Check sheet for the modelled part. Datum: model origin and axes. Units: mm. Coordinates: 2 decimals unless noted, no trailing zeros. Order: outer loops, then holes, each group sorted by start corner. A loop starts at its lowest first (then second) coordinate and runs counter-clockwise, first axis right, second up. Notation, with made-up numbers: M 59,88.25 L 80,88.25 A20 cw 80,116.25 Z; hole C 70,83.5 d7. An arc over 180 degrees is marked long. Answer in a Markdown table with one row per item. Add a question column.
Autodesk Fusion 360 part; units mm, degrees
sketch "Sketch1" plane through (0, 0, 0) normal (0, 0, 1) x (1, 0, 0)
  line L0 (-11.375, 11.375) -> (11.375, 11.375)
  line L1 (11.375, 11.375) -> (11.375, -11.375)
  line L2 (11.375, -11.375) -> (-11.375, -11.375)
  line L3 (-11.375, -11.375) -> (-11.375, 11.375)
  circle A0 centre (0, 0) radius 9
  point P0 (0, 11.375)
  point P1 (11.375, 0)
  dimension "d1" = 22.75
  dimension "d2" = 18
extrude "Extrude3" add sketch "Sketch1" along normal blind 9.75
1. Section check B-B on z = 1.75. Enter the section's corners in (x, y) (3 decimals).
2. Release check for a two-part mould opening along X. For faces 1 (the flat face through (11.375, 0, 5)), 2 (the flat face through (-11.375, 0, 5)), 3 (the cylindrical face through (-1.172, -8.923, 4.807)), 4 (the flat face through (0, -11.375, 5)) record: released by +X, released by -X, zero draft, split by the parting line, or undercut.
3. Scan lines: line 1 (Y direction, x = 0, z = 3) (3 decimals); line 2 (Y direction, x = -1.5, z = 0.5) (3 decimals); line 3 (X direction, y = -5, z = 0.75) (3 decimals). Record each from-to range of solid material in increasing order.
4. Section check A-A on y = 0. Enter the section's corners in (x, z) (3 decimals).
Result sheet:
| question | item | result |
|---|---|---|
| 1 | outline | M -11.375,-11.375 L 11.375,-11.375 L 11.375,11.375 L -11.375,11.375 Z; hole C 0,0 d18 |
| 2 | face 1 | released by +X |
| 2 | face 2 | released by -X |
| 2 | face 3 | undercut |
| 2 | face 4 | zero draft |
| 3 | line 1 | -11.375 to -9, 9 to 11.375 |
| 3 | line 2 | -11.375 to -8.874, 8.874 to 11.375 |
| 3 | line 3 | -11.375 to -7.483, 7.483 to 11.375 |
| 4 | outline | M -11.375,0 L -9,0 L -9,9.75 L -11.375,9.75 Z; M 9,0 L 11.375,0 L 11.375,9.75 L 9,9.75 Z |
